The model under review builds one solid part; all positions refer to its coordinate system, in mm. A direction names the side the tool comes from. Round coordinates to 2 decimals unless told otherwise and drop trailing zeros. Write each loop counter-clockwise with the first axis right and the second up, starting at its lowest first coordinate (ties: lowest second). Pieces come first, ordered by that corner, then holes.
Item 1: Machinability: for faces 4 (the face through (35, 25, -37)), 5 (the face through (63, 30, -33)), 6 (the face through (60, 26, -31)), 7 (the face through (6, 8, -15)), 8 (the face through (38, 20, -22)), which of the approach directions +Z, -Z, +X, -X, +Y, -Y give a long, thin tool a straight path to every point of the face, cutting with its end or side? Answer none if there is none.
Item 2: Add section C-C (z = -17.5). Give the boundary of the cut face in (x, y), plus the area to 3 significant figures.
Item 3: Clearance check with flat-ended pins moving along their axes: pin 1 Ø8 at (y, z) = (39.5, -29) entering from +X; pin 2 Ø13.5 at (x, z) = (62, -46) entering from -Y; pin 3 Ø4 at (x, z) = (36.5, -31) entering from +Y; pin 4 Ø4 at (y, z) = (-3, -26.5) entering from -X. State where each tip first meets the part, or that it passes through.
Item 4: Add section B-B (x = 27). Give the boundary of the cut face in (y, z), plus the area to 3 significant figures.
Item 5: Draft analysis for pull direction Y (two halves, no side actions). For faces 1 (the face through (20.7, 53.26, -3.27)), 2 (the face through (54.707, 4.31, -0.592)), 3 (the face through (38, 25, -30)), state which applies: +Y half, -Y half, draft (parallel to the pull), parting line (faces both ways), or undercut.
Item 6: Add section A-A (y = 10). Give the boundary of the cut face in (x, z), plus the area to 3 significant figures.
Item 7: Add section D-D (x = 60). State how many separate pieces and enclosed holes the cut face has, plus the area to 3 significant figures.
Item 8: To check wall thickness, follow L1, parallel to X at y = 28.6, z = -38; L2, parallel to Y at x = 40.5, z = -56.5; L3, parallel to Y at x = 12.5, z = -18. State the ranges of each line that lie inside material, in increasing order.
```python
from build123d import *

# Parameters (mm, degrees)
SKETCH1_W                = 40
SKETCH1_H                = 40
BOSS_EXTRUDE1_DEPTH      = 40
SKETCH2_W                = 25
SKETCH2_H                = 20
CUT_EXTRUDE1_DEPTH       = 40
CHAMFER1_SIZE            = 15
CUT_EXTRUDE2_DEPTH       = 15
CHAMFER2_SIZE            = 4
SKETCH4_R                = 2.6
CUT_EXTRUDE3_DEPTH       = 17
BOSS_EXTRUDE2_DEPTH      = 8
BOSS_EXTRUDE2_DEPTH_BACK = 40
SKETCH5_W                = 40
SKETCH5_H                = 8.5
SKETCH10_W               = 14
SKETCH10_H               = 10
CUT_EXTRUDE5_DEPTH       = 26
SKETCH8_R                = 5.6
CUT_EXTRUDE4_DEPTH       = 34
BOSS_EXTRUDE3_DEPTH      = 20
FILLET3_R                = 4
FILLET4_R                = 2
CHAMFER7_SIZE            = 25
CHAMFER8_SIZE            = 2
CHAMFER8_SIZE2           = 10
FILLET7_R                = 2
SKETCH14_W               = 40
SKETCH14_H               = 8.5
BOSS_EXTRUDE4_DEPTH      = 15
SKETCH16_W               = 40
SKETCH16_H               = 8.5
BOSS_EXTRUDE5_DEPTH      = 15
SKETCH12_R               = 11.1
CUT_EXTRUDE6_DEPTH       = 4.5
CUT_EXTRUDE7_START       = -7.5
SKETCH13_R               = 11.1
CUT_EXTRUDE7_DEPTH       = 7.5
SKETCH15_R               = 2.1
CUT_EXTRUDE8_DEPTH       = 10
CHAMFER10_SIZE           = 0.5
FILLET8_R                = 8
CUT_EXTRUDE9_DEPTH       = 10


with BuildPart() as part:
    # Sketch1 → Boss-Extrude1 (new body)
    with BuildSketch(Plane(origin=(0, 0, 0), x_dir=(1, 0, 0), z_dir=(0, 1, 0))):
        with Locations((20, 20)):
            Rectangle(SKETCH1_W, SKETCH1_H)
    extrude(amount=BOSS_EXTRUDE1_DEPTH)

    # Sketch2 → Cut-Extrude1 (cut)
    with BuildSketch(Plane(origin=(0, 40, 0), x_dir=(1, 0, 0), z_dir=(0, 1, 0))):
        with Locations((12.5, 30)):
            Rectangle(SKETCH2_W, SKETCH2_H)
    extrude(amount=-CUT_EXTRUDE1_DEPTH, mode=Mode.SUBTRACT)

    # Chamfer1
    chamfer1_edges = [part.edges().sort_by_distance(p)[0] for p in [
        (0, 20, 0),
    ]]
    chamfer(chamfer1_edges, length=CHAMFER1_SIZE)

    # Sketch3 → Cut-Extrude2 (cut)
    with BuildSketch(Plane.XY):
        Polygon((0, 10), (0, 15), (15, 15), (15, 5), (0, 5), align=None)
        Polygon((0, 30), (0, 25), (15, 25), (15, 35), (0, 35), align=None)
    extrude(amount=-CUT_EXTRUDE2_DEPTH, mode=Mode.SUBTRACT)

    # Chamfer2
    chamfer2_edges = [part.edges().sort_by_distance(p)[0] for p in [
        (15, 35, -7.5),
        (15, 25, -7.5),
        (15, 15, -7.5),
        (15, 5, -7.5),
    ]]
    chamfer(chamfer2_edges, length=CHAMFER2_SIZE)

    # Sketch4 → Cut-Extrude3 (cut)
    with BuildSketch(Plane.XY.offset(-15)):
        with Locations((8, 30)):
            Circle(SKETCH4_R)
        with Locations((8, 10)):
            Circle(SKETCH4_R)
    extrude(amount=-CUT_EXTRUDE3_DEPTH, mode=Mode.SUBTRACT)

    # Sketch5 → Boss-Extrude2 (add, two sides: drawn at the far end of the back side and taken through both)
    with BuildSketch(Plane(origin=(0, 0, -40), x_dir=(-1, 0, 0), z_dir=(0, 0, -1)).offset(-BOSS_EXTRUDE2_DEPTH_BACK)):
        with Locations((-60, 4.25)):
            Rectangle(SKETCH5_W, SKETCH5_H)
        with Locations((-60, 30.25)):
            Rectangle(SKETCH5_W, SKETCH5_H)
    extrude(amount=BOSS_EXTRUDE2_DEPTH + BOSS_EXTRUDE2_DEPTH_BACK)

    # Sketch10 → Cut-Extrude5 (cut)
    with BuildSketch(Plane(origin=(40, 0, 0), x_dir=(0, 0, -1), z_dir=(1, 0, 0))):
        with Locations((29, 20)):
            Rectangle(SKETCH10_W, SKETCH10_H)
    extrude(amount=-CUT_EXTRUDE5_DEPTH, mode=Mode.SUBTRACT)

    # Sketch8 → Cut-Extrude4 (cut)
    with BuildSketch(Plane(origin=(0, 32, 0), x_dir=(1, 0, 0), z_dir=(0, 1, 0))):
        with Locations(Location((60, 38, 0), (0, 0, 270))):
            Circle(SKETCH8_R)
    extrude(amount=-CUT_EXTRUDE4_DEPTH, mode=Mode.SUBTRACT)

    # Sketch9 → Boss-Extrude3 (add)
    with BuildSketch(Plane(origin=(40, 0, 0), x_dir=(0, 0, -1), z_dir=(1, 0, 0))):
        Polygon((0, 40), (0, 55), (4, 55), (20, 40), align=None)
        Polygon((0, 0), (0, -15), (4, -15), (20, 0), align=None)
    extrude(amount=-BOSS_EXTRUDE3_DEPTH)

    # Fillet3
    fillet3_edges = [part.edges().sort_by_distance(p)[0] for p in [
        (20, 55, -2),
        (40, 55, -2),
        (20, -15, -2),
        (40, -15, -2),
    ]]
    fillet(fillet3_edges, radius=FILLET3_R)

    # Fillet4
    fillet4_edges = [part.edges().sort_by_distance(p)[0] for p in [
        (32.5, 40, -40),
        (32.5, 0, -40),
    ]]
    fillet(fillet4_edges, radius=FILLET4_R)

    # Chamfer7
    chamfer7_edges = [part.edges().sort_by_distance(p)[0] for p in [
        (80, 4.25, 0),
        (80, 30.25, 0),
    ]]
    chamfer(chamfer7_edges, length=CHAMFER7_SIZE)

    # Chamfer8
    chamfer8_edges = [part.edges().sort_by_distance(p)[0] for p in [
        (40, 20, -36),
    ]]
    chamfer8_side = [part.faces().sort_by_distance(p)[0] for p in [
        (40, 16.5625, -17.75),
    ]]
    chamfer(chamfer8_edges, length=CHAMFER8_SIZE, length2=CHAMFER8_SIZE2, reference=chamfer8_side[0])

    # Fillet7
    fillet7_edges = [part.edges().sort_by_distance(p)[0] for p in [
        (27.5, 15, -36),
        (32.5, 15, -22),
        (32.5, 25, -22),
        (27.5, 25, -36),
        (35, 25, -37),
        (35, 15, -37),
    ]]
    fillet(fillet7_edges, radius=FILLET7_R)

    # Sketch14 → Boss-Extrude4 (add)
    with BuildSketch(Plane(origin=(0, 0, -48), x_dir=(-1, 0, 0), z_dir=(0, 0, -1))):
        with Locations((-60, 4.25)):
            Rectangle(SKETCH14_W, SKETCH14_H)
    extrude(amount=BOSS_EXTRUDE4_DEPTH)

    # Sketch16 → Boss-Extrude5 (add)
    with BuildSketch(Plane(origin=(0, 0, -48), x_dir=(-1, 0, 0), z_dir=(0, 0, -1))):
        with Locations((-60, 30.25)):
            Rectangle(SKETCH16_W, SKETCH16_H)
    extrude(amount=BOSS_EXTRUDE5_DEPTH)

    # Sketch12 → Cut-Extrude6 (cut)
    with BuildSketch(Plane(origin=(0, 34.5, 0), x_dir=(1, 0, 0), z_dir=(0, 1, 0))):
        with Locations(Location((60, 38, 0), (0, 0, 180))):
            Circle(SKETCH12_R)
    extrude(amount=-CUT_EXTRUDE6_DEPTH, mode=Mode.SUBTRACT)

    # Sketch13 → Cut-Extrude7 (cut)
    with BuildSketch(Plane.XZ.offset(CUT_EXTRUDE7_START)):
        with Locations(Location((60, -38, 0), (0, 0, 180))):
            Circle(SKETCH13_R)
    extrude(amount=CUT_EXTRUDE7_DEPTH, mode=Mode.SUBTRACT)

    # Sketch15 → Cut-Extrude8 (cut)
    with BuildSketch(Plane.XZ):
        with Locations(Location((60, -54.130501699, 0), (0, 0, 270))):
            Circle(SKETCH15_R)
        with Locations(Location((60, -21.869498301, 0), (0, 0, 270))):
            Circle(SKETCH15_R)
    extrude(amount=-CUT_EXTRUDE8_DEPTH, mode=Mode.SUBTRACT)

    # Chamfer10
    chamfer10_edges = [part.edges().sort_by_distance(p)[0] for p in [
        (71.1, 34.5, -38),
        (71.1, 0, -38),
    ]]
    chamfer(chamfer10_edges, length=CHAMFER10_SIZE)

    # Fillet8
    fillet8_edges = [part.edges().sort_by_distance(p)[0] for p in [
        (55, 30.25, 0),
        (55, 4.25, 0),
        (80, 4.25, -25),
        (80, 30.25, -25),
        (80, 4.25, -63),
        (40, 4.25, -63),
        (80, 30.25, -63),
        (40, 30.25, -63),
    ]]
    fillet(fillet8_edges, radius=FILLET8_R)

    # Sketch17 → Cut-Extrude9 (cut)
    with BuildSketch(Plane.ZY.offset(-25)):
        Polygon((-20, 0), (-20, 68.838193982), (-62.566783677, 68.838193982), (-62.566783677, -51.070720767), align=None)
    extrude(amount=-CUT_EXTRUDE9_DEPTH, mode=Mode.SUBTRACT)


solid = part.part
```
Numbers:
1. face 4: -Z, -X, +Y, -Y
1. face 5: +Y
1. face 6: +Z, -Z, +X
1. face 7: +Z, -X
1. face 8: +X, -X
2. outline: (0, 0) - (20, 0) - (20, -2.34) - (40, -2.34) - (40, 0) - (72.5, 0) - (72.5, 8.5) - (40, 8.5) - (40, 26) - (72.5, 26) - (72.5, 34.5) - (40, 34.5) - (40, 42.34) - (20, 42.34) - (20, 40) - (0, 40) - close; hole circle Ø5.2 at (8, 10); hole circle Ø5.2 at (8, 30)
2. area: 2,200 mm2
3. pin 1: stops at x = 40
3. pin 2: stops at y = 0
3. pin 3: stops at y = 40
3. pin 4: passes through
4. outline: (-15, -4) - (0, -20) - (40, -20) - (55, -4) - (55, 0) - (-15, 0) - close
4. area: 1,160 mm2
5. face 1: +Y half
5. face 2: draft
5. face 3: undercut
6. outline: (0, -20) - (5.4, -20) - (5.4, -15) - (0, -15) - close; (10.6, -20) - (35, -20) - (35, -40) - (40, -40) - (40, 0) - (15, 0) - (15, -15) - (10.6, -15) - close
6. area: 649 mm2
7. separate pieces: 6
7. enclosed holes: 0
7. area: 592 mm2
8. L1: x = 35 to 54.4, 65.6 to 80
8. L2: y = 0 to 8.5, 26 to 34.5
8. L3: y = 0 to 40
